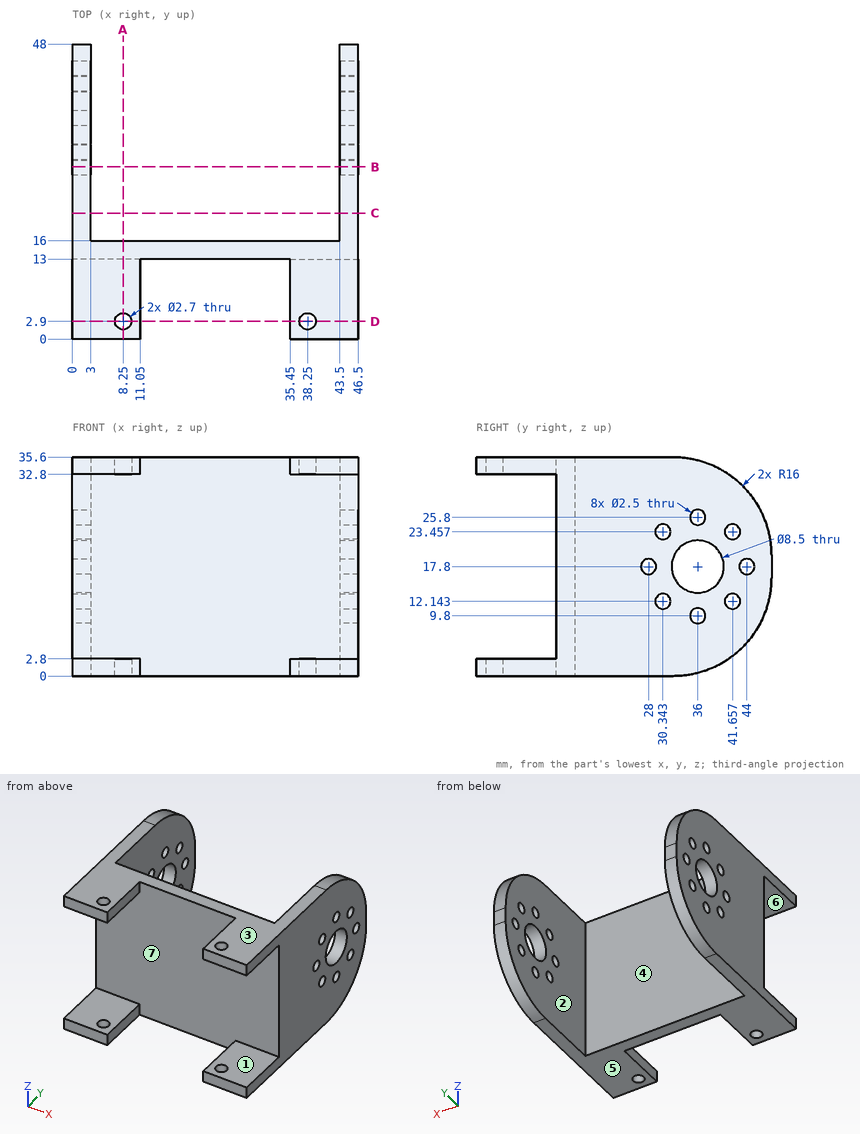
For this review, use the dimensioned drawing (mm, ordinates from the lowest corner) and the shaded views. A direction names the side the tool comes from. Round coordinates to 2 decimals unless told otherwise and drop trailing zeros. Order: outer loops, then holes, each group sorted by start corner. A loop starts at its lowest first (then second) coordinate and runs counter-clockwise, first axis right, second up. Notation, with made-up numbers: (5.5, 13.5) -> (26.5, 13.5) arc R16 cw to (26.5, 31.5) -> close; hole circle Ø9 at (75.5, 66.5). An arc over 180 degrees is marked (long way). Put each result on its own line as item: value.
Q1. Machinability: for the marked faces 1, 2 and 3, which of the approach directions +Z, -Z, +X, -X, +Y, -Y give a long, thin tool a straight path to every point of the face, cutting with its end or side? Answer none if there is none.
Check result:
face 1: +X, -X, -Y
face 2: +Z, -Z, +Y
face 3: +Z, +X, -X, +Y, -Y
Q2. Add section D-D on y = 2.9. State how many separate pieces and enclosed holes the cut face has.
Check result:
separate pieces: 8
enclosed holes: 0
Q3. For probe 1 along Y at (x, z) = (44.5, 17.8); probe 2 along Y at (x, z) = (8.25, 2.2); probe 3 along X at (y, z) = (25, 25), list the stretches that pass through material, from the lowest coordinate up. Write a range as [from, to].
Check result:
probe 1: [13, 26.75], [29.25, 31.75], [40.25, 42.75], [45.25, 48]
probe 2: [0, 1.55], [4.25, 16]
probe 3: [0, 3], [43.5, 46.5]
Q4. Insertion check: pin 1 Ø2 at (y, z) = (41.66, 12.14) entering from -X; pin 2 Ø5 at (x, z) = (41.5, 9.5) entering from +Y; pin 3 Ø11 at (y, z) = (36, 17.8) entering from -X; pin 4 Ø18 at (x, z) = (25, 22.5) entering from +Y. Each pin has a flat end and moves straight along its axis. Give the tip position at first contact, or say it passes through.
Check result:
pin 1: through
pin 2: y = 47.2
pin 3: x = 0
pin 4: y = 16
Q5. Add section C-C on y = 20.5. Write out the cut boundary in (x, z), plus the area to 3 significant figures.
Check result:
outline: (0, 0) -> (3, 0) -> (3, 35.6) -> (0, 35.6) -> close; (43.5, 0) -> (46.5, 0) -> (46.5, 35.6) -> (43.5, 35.6) -> close
area: 214 mm2
Q6. Add section B-B on y = 28. Write out the cut boundary in (x, z).
Check result:
outline: (0, 0) -> (3, 0) -> (3, 16.55) -> (0, 16.55) -> close; (0, 19.05) -> (3, 19.05) -> (3, 35.6) -> (0, 35.6) -> close; (43.5, 0) -> (46.5, 0) -> (46.5, 16.55) -> (43.5, 16.55) -> close; (43.5, 19.05) -> (46.5, 19.05) -> (46.5, 35.6) -> (43.5, 35.6) -> close
Q7. Mouldability with a two-part tool opening along Z and no side actions: class the marked faces 4, 5, 6 and 7 as pulls with the +Z half, pulls with the -Z half, needs draft (parallel to the pull), parting line crosses it, or undercut.
Check result:
face 4: needs draft
face 5: pulls with the -Z half
face 6: undercut
face 7: undercut
Q8. Add section A-A on x = 8.25. Write out the cut boundary in (y, z).
Check result:
outline: (0, 0) -> (1.55, 0) -> (1.55, 2.8) -> (0, 2.8) -> close; (0, 32.8) -> (1.55, 32.8) -> (1.55, 35.6) -> (0, 35.6) -> close; (4.25, 0) -> (16, 0) -> (16, 35.6) -> (4.25, 35.6) -> (4.25, 32.8) -> (13, 32.8) -> (13, 2.8) -> (4.25, 2.8) -> close
